The model under review builds one solid part; all positions refer to its coordinate system, in mm. Face numbers are marked on the shaded views. A direction names the side the tool comes from. Coordinates: 2 decimals unless noted, no trailing zeros. Write each loop counter-clockwise with the first axis right and the second up, starting at its lowest first coordinate (ties: lowest second). Pieces come first, ordered by that corner, then holes. Notation, with made-up numbers: (26.25, 4) - (51.25, 4) arc R17 ccw to (51.25, 36) - close; hole circle Ø8 at (72.5, 74.5). An arc over 180 degrees is marked (long way). Return JSON: item names as keys, results as strings. Group by question number.
(1) We need section D-D on x = 3. State the section outline as (y, z) points, then the cut area to 3 significant figures.
(2) Tool access review of the marked faces 3, 4 and 5: name each direction out of +Z, -Z, +X, -X, +Y, -Y from which nothing blocks a thin tool from reaching the whole face with its end or side.
(3) We need section C-C on z = 13. State the section outline as (x, y) points.
(4) For pin 1 Ø1 at (y, z) = (-1, 21.5) entering from -X; pin 2 Ø1.5 at (x, y) = (1, 1.5) entering from +Z; pin 3 Ø1.5 at (x, z) = (-2, 26.5) entering from -Y, all flat-tipped, find the tip position at first contact; note any pin that passes through.
(5) Draft analysis for pull direction X (two halves, no side actions). For the marked faces 1 and 2, state which applies: released by +X, released by -X, zero draft, split by the parting line, or undercut.
(6) We need section A-A on x = 0. State the section outline as (y, z) points, then the cut area to 3 significant figures.
(7) To check wall thickness, follow L1, parallel to Z at x = 0.25, y = 1.5; L2, parallel to Z at x = 0.5, y = -2.5; L3, parallel to Y at x = -2, z = 5.5. State the ranges of each line that lie inside material, in increasing order. Write a range as from..to.
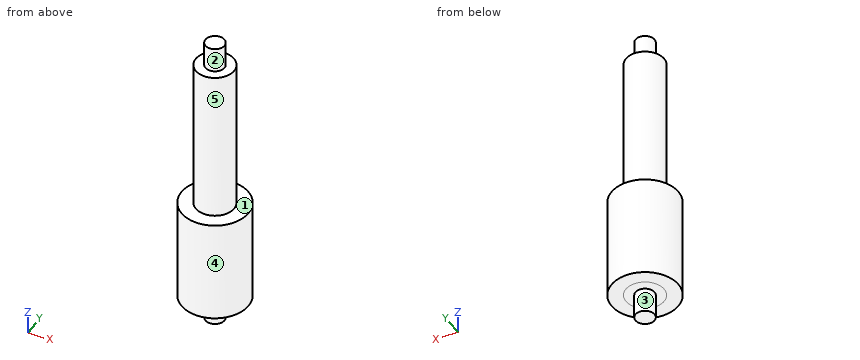
```python
from build123d import *

# Parameters (mm, degrees)
EXTRUDE_START   = 3.386462
SKETCH_1_R      = 2
EXTRUDE_1_DEPTH = 27.013538
SKETCH_2_R      = 1
EXTRUDE_2_DEPTH = 2.6
SKETCH_4_R      = 1
EXTRUDE_3_DEPTH = 2.6
EXTRUDE_START_2 = -10.863538
SKETCH_6_R      = 3.5
EXTRUDE_5_DEPTH = 10.863538


with BuildPart() as part:
    # Эскиз1 → Бобышка-Вытянуть1 (new body)
    with BuildSketch(Plane.XY.offset(EXTRUDE_START)):
        Circle(SKETCH_1_R)
    extrude(amount=EXTRUDE_1_DEPTH)

    # Эскиз2 → Бобышка-Вытянуть2 (add)
    with BuildSketch(Plane.XY.offset(30.4)):
        Circle(SKETCH_2_R)
    extrude(amount=EXTRUDE_2_DEPTH)

    # Эскиз4 → Бобышка-Вытянуть3 (add)
    with BuildSketch(Plane(origin=(0, 0, 3.386462289), x_dir=(-1, 0, 0), z_dir=(0, 0, -1))):
        Circle(SKETCH_4_R)
    extrude(amount=EXTRUDE_3_DEPTH)

    # Эскиз6 → Бобышка-Вытянуть5 (add)
    with BuildSketch(Plane(origin=(0, 0, 3.386462289), x_dir=(-1, 0, 0), z_dir=(0, 0, -1)).offset(EXTRUDE_START_2)):
        Circle(SKETCH_6_R)
    extrude(amount=EXTRUDE_5_DEPTH)


solid = part.part
```
Ans:
{
 "1": {"outline": "(-1.8, 3.39) - (1.8, 3.39) - (1.8, 14.25) - (-1.8, 14.25) - close", "area": "39.2 mm²"},
 "2": {"face 3": "-Z", "face 4": "+Z, -Z", "face 5": "+Z"},
 "3": {"outline": "circle Ø7 at (0, 0)"},
 "4": {"pin 1": "x = -1.94", "pin 2": "z = 30.4", "pin 3": "y = -1.56"},
 "5": {"face 1": "zero draft", "face 2": "split by the parting line"},
 "6": {"outline": "(-3.5, 3.39) - (-1, 3.39) - (-1, 0.79) - (1, 0.79) - (1, 3.39) - (3.5, 3.39) - (3.5, 14.25) - (2, 14.25) - (2, 30.4) - (1, 30.4) - (1, 33) - (-1, 33) - (-1, 30.4) - (-2, 30.4) - (-2, 14.25) - (-3.5, 14.25) - close", "area": "151 mm²"},
 "7": {"L1": "3.39..30.4", "L2": "3.39..14.25", "L3": "-2.87..2.87"}
}
